```python
from build123d import *

# Parameters (mm, degrees)
F1_DEPTH = 19.05


with BuildPart() as f1:
    # F0 (on Right) → F1 (new body)
    with BuildSketch(Plane.YZ):
        with BuildLine():
            Line((131.826, -158.75), (131.826, 158.75))
            Line((131.826, 158.75), (12.7, 158.75))
            Line((12.7, 158.75), (12.7, 146.05))
            ThreePointArc((12.7, 146.05), (0, 133.35), (-12.7, 146.05))
            Line((-12.7, 146.05), (-12.7, 158.75))
            Line((-12.7, 158.75), (-131.826, 158.75))
            Line((-131.826, 158.75), (-131.826, -158.75))
            Line((-131.826, -158.75), (131.826, -158.75))
        make_face()
    extrude(amount=F1_DEPTH)


solid = f1.part
```
Geometry: final body of the model. Coordinates: model frame, mm. A direction names the side the tool comes from. Round coordinates to 2 decimals unless told otherwise and drop trailing zeros. Order: outer loops, then holes, each group sorted by start corner. A loop starts at its lowest first (then second) coordinate and runs counter-clockwise, first axis right, second up. Notation, with made-up numbers: (42.25, 62) -> (84.25, 62) arc R29 cw to (84.25, 85) -> close; hole circle Ø3 at (44.25, 83). An arc over 180 degrees is marked (long way). Use CSV: the item, a comma, the result in double quotes. Start each with the question number.
1) Draft query along Y for faces 1 (the face through (9, 12.7, 152)), 2 (the face through (9, 73, 158.75)), 3 (the face through (9, 131.826, -2)). Return one class per face: +Y half, -Y half, draft (parallel to the pull), parting line (faces both ways), or undercut.
2) Section A-A (y = 0). Return the cut outline in (x, z), and give its area (3 significant figures).
3) First-contact query: pin 1 Ø3 at (y, z) = (34.5, -96) entering from -X. Flat tip, straight axial feed; report the tip coordinate or a pass-through.
4) Set-up query: faces 4 (the face through (9, -12.7, 152)), 5 (the face through (9, -71, 158.75)). Return all of +Z, -Z, +X, -X, +Y, -Y with unobstructed straight access to the full face (end or side cutting, diameter ignored); none if empty.
5) Material intervals for line 1 along Z through (x, y) = (15, -11.5); line 2 along Z through (x, y) = (8.5, 11), sorted ascending. Write a range as from..to.
Returned:
1,face 1,"undercut"
1,face 2,"draft"
1,face 3,"+Y half"
2,outline,"(0, -158.75) -> (19.05, -158.75) -> (19.05, 133.35) -> (0, 133.35) -> close"
2,area,"5,560 mm²"
3,pin 1,"stops at x = 0"
4,face 4,"+Z, +X, -X"
4,face 5,"+Z, +X, -X, +Y, -Y"
5,line 1,"z = -158.75..140.66"
5,line 2,"z = -158.75..139.7"
